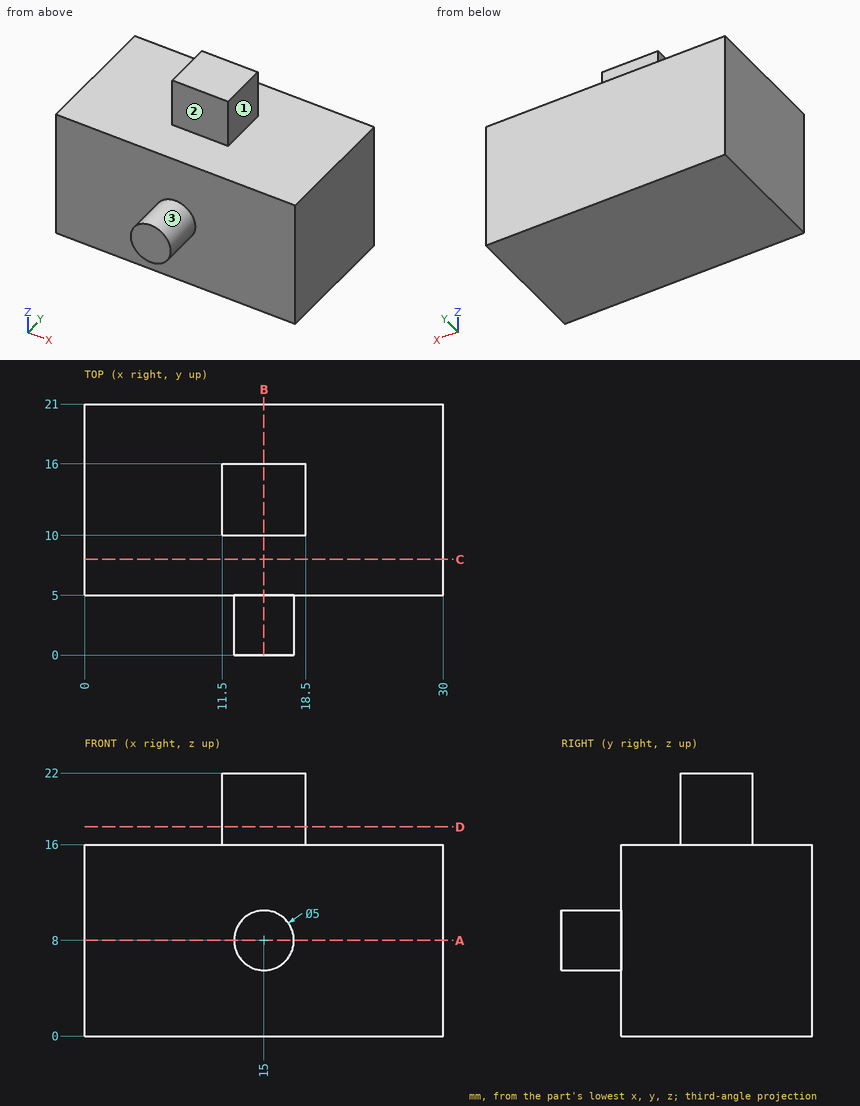
Drawing for the job (mm, zero at the part's lowest x, y, z). A direction names the side the tool comes from. Give positions to 0.01 mm unless a question says otherwise; leave off trailing zeros. Write each loop counter-clockwise with the first axis right and the second up, starting at its lowest first coordinate (ties: lowest second). Pieces come first, ordered by that corner, then holes. Notation, with made-up numbers: M 37.25,41.5 L 57.25,41.5 A18 cw 57.25,50.5 Z; hole C 88.25,-15.5 d2. An arc over 180 degrees is marked long. Return JSON: item names as keys, results as strings. Group by question number.
(1) Flat gauge pins, fed straight in: pin 1 Ø4 at (x, z) = (21, 6) entering from -Y; pin 2 Ø5 at (y, z) = (13, 19.5) entering from -X; pin 3 Ø1.8 at (x, z) = (14, 20) entering from -Y. Where does each tip first touch, or does it go through?
(2) Band-saw the part on C-C (y = 8). Give the cut face in (x, z), and give its area (3 significant figures).
(3) Band-saw the part on B-B (x = 15). Give the cut face in (y, z), and give its area (3 significant figures).
(4) Band-saw the part on A-A (z = 8). Give the cut face in (x, y), and give its area (3 significant figures).
(5) Band-saw the part on D-D (z = 17.5). Give the cut face in (x, y), and give its area (3 significant figures).
(6) Drill centre lines: L1, parallel to Z at x = 11, y = 14.5; L2, parallel to Y at x = 12, z = 8.5; L3, parallel to X at y = 11.5, z = 20. Where is each one in solid material? Low to high. Write a range as [from, to].
(7) 3-axis set-ups, long thin cutter, end or side, ignore diameter. For the marked faces 1, 2 and 3: which of +Z, -Z, +X, -X, +Y, -Y reach the whole face in a straight line?
Entries:
{
 "1": {"pin 1": "stops at y = 5", "pin 2": "stops at x = 11.5", "pin 3": "stops at y = 10"},
 "2": {"outline": "M 0,0 L 30,0 L 30,16 L 0,16 Z", "area": "480 mm^2"},
 "3": {"outline": "M 0,5.5 L 5,5.5 L 5,0 L 21,0 L 21,16 L 16,16 L 16,22 L 10,22 L 10,16 L 5,16 L 5,10.5 L 0,10.5 Z", "area": "317 mm^2"},
 "4": {"outline": "M 0,5 L 12.5,5 L 12.5,0 L 17.5,0 L 17.5,5 L 30,5 L 30,21 L 0,21 Z", "area": "505 mm^2"},
 "5": {"outline": "M 11.5,10 L 18.5,10 L 18.5,16 L 11.5,16 Z", "area": "42.0 mm^2"},
 "6": {"L1": "z = [0, 16]", "L2": "y = [5, 21]", "L3": "x = [11.5, 18.5]"},
 "7": {"face 1": "+Z, +X, +Y, -Y", "face 2": "+Z, +X, -X, -Y", "face 3": "-Y"}
}
